Input: part model. Units: mm. Frame: model coordinates. A direction names the side the tool comes from. Give positions to 0.01 mm unless a question says otherwise; leave off trailing zeros. Write each loop counter-clockwise with the first axis right and the second up, starting at its lowest first coordinate (ties: lowest second). Pieces come first, ordered by that corner, then holes. Notation, with made-up numbers: (-13, 9) -> (29, 9) arc R24 ccw to (29, 33) -> close; hole circle Ø11 at (7.5, 15). An arc over 180 degrees is marked (long way). Return JSON: item names as keys, results as strings. Group by question number.
Item 1: Section A-A, the plane x = 0. Return loops of the section in (y, z), then the cut area to 3 significant figures.
Item 2: Section D-D, the plane y = -5. Return loops of the section in (x, z).
Item 3: Pin query (flat end, axial travel): P1, Ø1.8, axis at x = -19.5, y = -5, coming from the +Z side; P2, Ø4, axis at x = -5, z = 3.5, coming from the -Y side; P3, Ø12, axis at x = -8.5, y = -7.5, coming from the +Z side. Return the tip coordinate at first contact, or that it passes through.
Item 4: Set-up query: faces 4 (the face through (19.3, 3.7, 3.8)), 5 (the face through (-19.31, 4, 1.87)), 6 (the face through (-20.5, -9.53, 1.23)). Return all of +Z, -Z, +X, -X, +Y, -Y with unobstructed straight access to the full face (end or side cutting, diameter ignored); none if empty.
Item 5: Line query: line 1 (Y direction, x = 18, z = 5.7); line 2 (Y direction, x = -17, z = 6.75); line 3 (Y direction, x = 0, z = 2.55). Output: solid intervals per line, ascending. Write a range as [from, to].
Item 6: Section B-B, the plane y = 0. Return loops of the section in (x, z), then the cut area to 3 significant figures.
Item 7: Section C-C, the plane z = 3.25. Return loops of the section in (x, y).
Item 8: Mould query, pull axis X, two halves, no side actions, for faces 1 (the face through (0, 12, 3)), 2 (the face through (21.217, 8.147, 3.451)), 3 (the face through (20, -9.5, 7.7)). Classes: released by +X, released by -X, zero draft, split by the parting line, or undercut.
from build123d import *

# Parameters (mm, degrees)
SKETCH2_R           = 1.65
BOSS_EXTRUDE1_DEPTH = 7
SKETCH3_R           = 9.7
CUT_EXTRUDE1_DEPTH  = 5
SKETCH4_R           = 7.5
CUT_EXTRUDE2_DEPTH  = 5
CUT_EXTRUDE3_DEPTH  = 2.5
SKETCH8_R           = 2.95
CUT_EXTRUDE4_DEPTH  = 3.2
SKETCH9_R           = 2.5
SKETCH9_R_2         = 1.65
BOSS_EXTRUDE2_DEPTH = 1.5
MOVE_FACE1_BY       = 0.5


with BuildPart() as part:
    # Sketch2 → Boss-Extrude1 (new body)
    with BuildSketch(Plane.XY):
        with BuildLine():
            Line((-7.331439149, 9.5), (-18, 9.5))
            ThreePointArc((-18, 9.5), (-21.181980515, 8.181980515), (-22.5, 5))
            Line((-22.5, 5), (-22.5, -11))
            ThreePointArc((-22.5, -11), (-19.789453748, -15.128904853), (-14.92317543, -14.283770784))
            ThreePointArc((-14.92317543, -14.283770784), (-9.507484415, -11.369138817), (-3.359154955, -11.520246438))
            ThreePointArc((-3.359154955, -11.520246438), (0, -12), (3.359154955, -11.520246438))
            ThreePointArc((3.359154955, -11.520246438), (9.507484415, -11.369138817), (14.92317543, -14.283770784))
            ThreePointArc((14.92317543, -14.283770784), (19.789453748, -15.128904853), (22.5, -11))
            Line((22.5, -11), (22.5, 5))
            ThreePointArc((22.5, 5), (21.181980515, 8.181980515), (18, 9.5))
            Line((18, 9.5), (7.331439149, 9.5))
            ThreePointArc((7.331439149, 9.5), (0, 12), (-7.331439149, 9.5))
        make_face()
        with Locations((-18, 5)):
            Circle(SKETCH2_R, mode=Mode.SUBTRACT)
        with Locations((-18, -11)):
            Circle(SKETCH2_R, mode=Mode.SUBTRACT)
        with Locations((-18, -5)):
            Circle(SKETCH2_R, mode=Mode.SUBTRACT)
        with Locations(Location((18, -5, 0), (0, 0, 180))):
            Circle(SKETCH2_R, mode=Mode.SUBTRACT)
        with Locations(Location((18, -11, 0), (0, 0, 180))):
            Circle(SKETCH2_R, mode=Mode.SUBTRACT)
        with Locations(Location((18, 5, 0), (0, 0, 180))):
            Circle(SKETCH2_R, mode=Mode.SUBTRACT)
    extrude(amount=BOSS_EXTRUDE1_DEPTH)

    # Sketch3 → Cut-Extrude1 (cut)
    with BuildSketch(Plane.XY):
        Circle(SKETCH3_R)
    extrude(amount=CUT_EXTRUDE1_DEPTH, mode=Mode.SUBTRACT)

    # Sketch4 → Cut-Extrude2 (cut)
    with BuildSketch(Plane(origin=(0, 0, 5), x_dir=(-1, 0, 0), z_dir=(0, 0, -1))):
        Circle(SKETCH4_R)
    extrude(amount=-CUT_EXTRUDE2_DEPTH, mode=Mode.SUBTRACT)

    # Sketch6 → Cut-Extrude3 (cut)
    with BuildSketch(Plane(origin=(0, 0, 0), x_dir=(-1, 0, 0), z_dir=(0, 0, -1))):
        Polygon((-16.325684219, -8.1), (-19.674315781, -8.1), (-21.348631561, -11), (-19.674315781, -13.9), (-16.325684219, -13.9), (-14.651368439, -11), align=None)
        Polygon((14.651368439, -11), (16.325684219, -8.1), (19.674315781, -8.1), (21.348631561, -11), (19.674315781, -13.9), (16.325684219, -13.9), align=None)
    extrude(amount=-CUT_EXTRUDE3_DEPTH, mode=Mode.SUBTRACT)

    # Sketch8 → Cut-Extrude4 (cut)
    with BuildSketch(Plane.XY.offset(7)):
        with Locations((18, -5)):
            Circle(SKETCH8_R)
        with Locations((18, 5)):
            Circle(SKETCH8_R)
        with Locations((-18, 5)):
            Circle(SKETCH8_R)
        with Locations((-18, -5)):
            Circle(SKETCH8_R)
    extrude(amount=-CUT_EXTRUDE4_DEPTH, mode=Mode.SUBTRACT)

    # Sketch9 → Boss-Extrude2 (add)
    with BuildSketch(Plane.XY.offset(7)):
        with Locations((-18, -11)):
            Circle(SKETCH9_R)
        with Locations((-18, -11)):
            Circle(SKETCH9_R_2, mode=Mode.SUBTRACT)
        with Locations(Location((18, -11, 0), (0, 0, 180))):
            Circle(SKETCH9_R)
        with Locations(Location((18, -11, 0), (0, 0, 180))):
            Circle(SKETCH9_R_2, mode=Mode.SUBTRACT)
    extrude(amount=BOSS_EXTRUDE2_DEPTH)

    # Move Face1: a face moved outward by 0.5
    extrude(part.faces().sort_by_distance((-18, -13, 8.5))[0], amount=MOVE_FACE1_BY, dir=(0, 0, 1))


solid = part.part
Answer below:
{
 "1": {"outline": "(-12, 0) -> (-9.7, 0) -> (-9.7, 5) -> (-7.5, 5) -> (-7.5, 7) -> (-12, 7) -> close; (7.5, 5) -> (9.7, 5) -> (9.7, 0) -> (12, 0) -> (12, 7) -> (7.5, 7) -> close", "area": "41.0 mm2"},
 "2": {"outline": "(-22.5, 0) -> (-19.65, 0) -> (-19.65, 3.8) -> (-20.95, 3.8) -> (-20.95, 7) -> (-22.5, 7) -> close; (-16.35, 0) -> (-8.31, 0) -> (-8.31, 5) -> (-5.59, 5) -> (-5.59, 7) -> (-15.05, 7) -> (-15.05, 3.8) -> (-16.35, 3.8) -> close; (5.59, 5) -> (8.31, 5) -> (8.31, 0) -> (16.35, 0) -> (16.35, 3.8) -> (15.05, 3.8) -> (15.05, 7) -> (5.59, 7) -> close; (19.65, 0) -> (22.5, 0) -> (22.5, 7) -> (20.95, 7) -> (20.95, 3.8) -> (19.65, 3.8) -> close"},
 "3": {"P1": "stops at z = 3.8", "P2": "stops at y = -11.62", "P3": "stops at z = 7"},
 "4": {"face 4": "+Z", "face 5": "+Z, -Z", "face 6": "-Z"},
 "5": {"line 1": "y = [-15.5, -12.65], [-9.35, -7.95], [-2.05, 2.05], [7.95, 9.5]", "line 2": "y = [-15.39, -12.31], [-9.69, -7.78], [-2.22, 2.22], [7.78, 9.5]", "line 3": "y = [-12, -9.7], [9.7, 12]"},
 "6": {"outline": "(-22.5, 0) -> (-9.7, 0) -> (-9.7, 5) -> (-7.5, 5) -> (-7.5, 7) -> (-22.5, 7) -> close; (7.5, 5) -> (9.7, 5) -> (9.7, 0) -> (22.5, 0) -> (22.5, 7) -> (7.5, 7) -> close", "area": "188 mm2"},
 "7": {"outline": "(-22.5, -11) arc R4.5 ccw to (-14.92, -14.28) arc R12 cw to (-3.36, -11.52) arc R12 ccw to (3.36, -11.52) arc R12 cw to (14.92, -14.28) arc R4.5 ccw to (22.5, -11) -> (22.5, 5) arc R4.5 ccw to (18, 9.5) -> (7.33, 9.5) arc R12 ccw to (-7.33, 9.5) -> (-18, 9.5) arc R4.5 ccw to (-22.5, 5) -> close; hole circle Ø3.3 at (-18, -11); hole circle Ø3.3 at (-18, -5); hole circle Ø3.3 at (-18, 5); hole circle Ø19.4 at (0, 0); hole circle Ø3.3 at (18, -11); hole circle Ø3.3 at (18, -5); hole circle Ø3.3 at (18, 5)"},
 "8": {"face 1": "split by the parting line", "face 2": "released by +X", "face 3": "undercut"}
}
